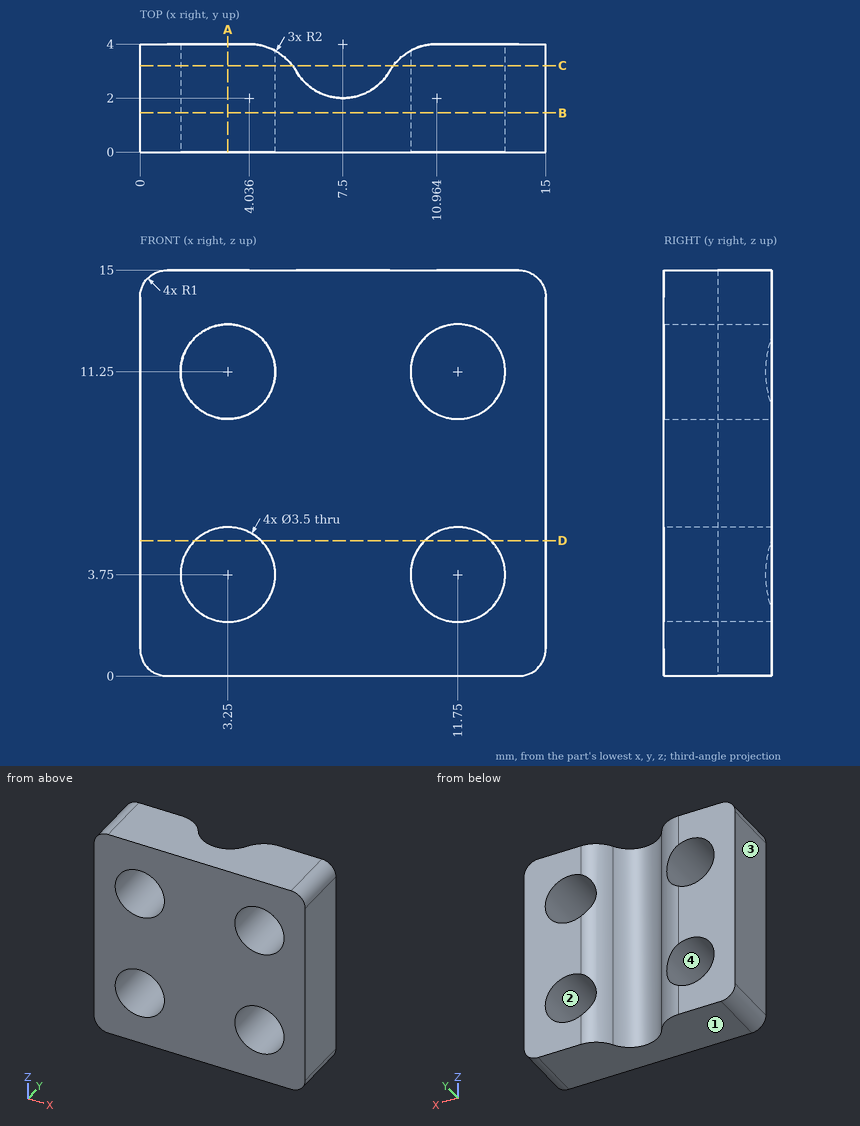
Input: dimensioned drawing with shaded views. Units: mm. Origin: part minimum x, y, z. Coordinates: 2 decimals unless noted, no trailing zeros. Order: outer loops, then holes, each group sorted by start corner. A loop starts at its lowest first (then second) coordinate and runs counter-clockwise, first axis right, second up.
Item 1: Draft query along X for the marked faces 1, 2, 3 and 4. Return one class per face: released by +X, released by -X, zero draft, split by the parting line, or undercut.
Answer:
face 1: zero draft
face 2: undercut
face 3: released by -X
face 4: undercut
Item 2: Section query A-A (x = 3.25). Output: boundary loops of the cut face in (y, z), then the cut area to 3 significant figures.
Answer:
outline: (0, 0) - (4, 0) - (4, 2) - (0, 2) - close; (0, 5.5) - (4, 5.5) - (4, 9.5) - (0, 9.5) - close; (0, 13) - (4, 13) - (4, 15) - (0, 15) - close
area: 32.0 mm2
Item 3: Contact query for flat-ended pins moving along their axis: P1, Ø3, axis at x = 11.5, z = 3.5, coming from the +Y side; P2, Ø2, axis at x = 3.25, z = 3.75, coming from the +Y side. Output: stop coordinate, or through.
Answer:
P1: stops at y = 4
P2: passes through
Item 4: Section query C-C (y = 3.2). Output: boundary loops of the cut face in (x, z).
Answer:
outline: (0, 1) arc R1 ccw to (1, 0) - (5.64, 0) - (5.64, 15) - (1, 15) arc R1 ccw to (0, 14) - close; (9.36, 0) - (14, 0) arc R1 ccw to (15, 1) - (15, 14) arc R1 ccw to (14, 15) - (9.36, 15) - close; hole circle Ø3.5 at (3.25, 3.75); hole circle Ø3.5 at (3.25, 11.25); hole circle Ø3.5 at (11.75, 3.75); hole circle Ø3.5 at (11.75, 11.25)
Item 5: Section query D-D (z = 5). Output: boundary loops of the cut face in (x, y), then the cut area to 3 significant figures.
Answer:
outline: (0, 0) - (2.03, 0) - (2.03, 4) - (0, 4) - close; (4.47, 0) - (10.53, 0) - (10.53, 3.95) arc R2 ccw to (9.23, 3) arc R2 cw to (5.77, 3) arc R2 ccw to (4.47, 3.95) - close; (12.97, 0) - (15, 0) - (15, 4) - (12.97, 4) - close
area: 33.5 mm2
Item 6: Section query B-B (y = 1.45). Output: boundary loops of the cut face in (x, z), then the cut area to 3 significant figures.
Answer:
outline: (0, 1) arc R1 ccw to (1, 0) - (14, 0) arc R1 ccw to (15, 1) - (15, 14) arc R1 ccw to (14, 15) - (1, 15) arc R1 ccw to (0, 14) - close; hole circle Ø3.5 at (3.25, 3.75); hole circle Ø3.5 at (3.25, 11.25); hole circle Ø3.5 at (11.75, 3.75); hole circle Ø3.5 at (11.75, 11.25)
area: 186 mm2
Item 7: Material intervals for line 1 along Z through (x, y) = (11.75, 3.5); line 2 along Z through (x, y) = (11.25, 3.55); line 3 along X through (y, z) = (0.9, 4.5), sorted ascending.
Answer:
line 1: z = 0 to 2, 5.5 to 9.5, 13 to 15
line 2: z = 0 to 2.07, 5.43 to 9.57, 12.93 to 15
line 3: x = 0 to 1.67, 4.83 to 10.17, 13.33 to 15
